Build history of the part. All positions in model axes, mm. A direction names the side the tool comes from. Round coordinates to 2 decimals unless told otherwise and drop trailing zeros. Write each loop counter-clockwise with the first axis right and the second up, starting at its lowest first coordinate (ties: lowest second). Pieces come first, ordered by that corner, then holes. Notation, with made-up numbers: (25.25, -0.75) -> (36.25, -0.75) arc R11 ccw to (36.25, 15.25) -> close; hole circle Ø8 at (83, 35). An arc over 180 degrees is marked (long way). Return JSON: item names as keys, results as strings.
from build123d import *

# Parameters (mm, degrees)
BASE_SKETCH_W                   = 20.493901532
BASE_SKETCH_H                   = 8
BASE_EXTRUDE_DEPTH              = 1.5
PROTRUSION_START                = 1.5
PROTRUSION_SKETCH_R             = 3
PROTRUSION_EXTRUDE_DEPTH        = 5
F_2_8_2_8_DIAMETER_HOLE1_D      = 2.8
PROTRUSION_CHAMFER_SIZE         = 0.25
F_2_5MM_DOWEL_HOLE3_D           = 2.5
F_2_5MM_DOWEL_HOLE3_DEPTH       = 6.5
F_2_5MM_DOWEL_HOLE3_CSINK_D     = 4
F_2_5MM_DOWEL_HOLE3_CSINK_ANGLE = 60
F_5MM_CIRCLE_SKETCH_R           = 2.5
F_5MM_DIAMETER_CUT_DEPTH        = 0.7


with BuildPart() as part:
    # Base Sketch → Base Extrude (new body)
    with BuildSketch(Plane(origin=(0, 0, 0), x_dir=(1, 0, 0), z_dir=(0, 1, 0))):
        with BuildLine():
            Line((-10.246950766, -4), (-10.246950766, 4))
            ThreePointArc((-10.246950766, 4), (-11, 0), (-10.246950766, -4))
        make_face()
        Rectangle(BASE_SKETCH_W, BASE_SKETCH_H)
        with BuildLine():
            Line((10.246950766, -4), (10.246950766, 4))
            ThreePointArc((10.246950766, 4), (11, 0), (10.246950766, -4))
        make_face()
    extrude(amount=BASE_EXTRUDE_DEPTH)

    # Protrusion Sketch → Protrusion Extrude (add)
    with BuildSketch(Plane(origin=(0, 0, 0), x_dir=(1, 0, 0), z_dir=(0, 1, 0)).offset(PROTRUSION_START)):
        Circle(PROTRUSION_SKETCH_R)
    extrude(amount=PROTRUSION_EXTRUDE_DEPTH)

    # Ø2.8 (2.8) Diameter Hole1 (through all)
    with Locations(Plane(origin=(0, 1.5, 0), x_dir=(1, 0, 0), z_dir=(0, 1, 0))):
        with Locations((-6.5, 0), (6.5, 0)):
            Hole(F_2_8_2_8_DIAMETER_HOLE1_D / 2)

    # Protrusion Chamfer
    protrusion_chamfer_edges = [part.edges().sort_by_distance(p)[0] for p in [
        (-3, 6.5, 0),
    ]]
    chamfer(protrusion_chamfer_edges, length=PROTRUSION_CHAMFER_SIZE)

    # Ø2.5mm Dowel Hole3
    with Locations(Plane(origin=(0, 6.5, 0), x_dir=(1, 0, 0), z_dir=(0, 1, 0))):
        with Locations((0, 0)):
            CounterSinkHole(F_2_5MM_DOWEL_HOLE3_D / 2, F_2_5MM_DOWEL_HOLE3_CSINK_D / 2, depth=F_2_5MM_DOWEL_HOLE3_DEPTH, counter_sink_angle=F_2_5MM_DOWEL_HOLE3_CSINK_ANGLE)

    # 5mm Circle Sketch → 5mm Diameter Cut (cut)
    with BuildSketch(Plane(origin=(0, 0, 0), x_dir=(1, 0, 0), z_dir=(0, 1, 0))):
        Circle(F_5MM_CIRCLE_SKETCH_R)
    extrude(amount=F_5MM_DIAMETER_CUT_DEPTH, mode=Mode.SUBTRACT)


solid = part.part
Q1. Saw through at A-A on x = -6.5. List the corners of the cut face in (y, z).
Verdict:
{"outline": "(0, -4) -> (1.5, -4) -> (1.5, -1.4) -> (0, -1.4) -> close; (0, 1.4) -> (1.5, 1.4) -> (1.5, 4) -> (0, 4) -> close"}
Q2. 3-axis set-ups, long thin cutter, end or side, ignore diameter. For faces 1 (the flat face through (-1, 0.7, 1)), 2 (the flat face through (-3, 0, 0)): which of +Z, -Z, +X, -X, +Y, -Y reach the whole face in a straight line?
Verdict:
{"face 1": "-Y", "face 2": "+Z, -Z, +X, -X, -Y"}
Q3. Pin check, flat tips, straight feed: pin 1 Ø1 at (y, z) = (3, -2.5) entering from +X; pin 2 Ø1.5 at (y, z) = (3, 2) entering from +X; pin 3 Ø3 at (y, z) = (1.5, -2) entering from -X. Stop position of each tip, or through.
Verdict:
{"pin 1": "stops at x = 2.24", "pin 2": "stops at x = 2.73", "pin 3": "stops at x = -10.99"}
Q4. Saw through at D-D on x = 0. List the corners of the cut face in (y, z), then the cut area to 3 significant figures.
Verdict:
{"outline": "(0, -4) -> (1.5, -4) -> (1.5, -3) -> (6.25, -3) -> (6.5, -2.75) -> (6.5, -2) -> (5.2, -1.25) -> (0.7, -1.25) -> (0.7, -2.5) -> (0, -2.5) -> close; (0, 2.5) -> (0.7, 2.5) -> (0.7, 1.25) -> (5.2, 1.25) -> (6.5, 2) -> (6.5, 2.75) -> (6.25, 3) -> (1.5, 3) -> (1.5, 4) -> (0, 4) -> close", "area": "23.0 mm²"}
Q5. Saw through at B-B on z = 0. List the corners of the cut face in (x, y), then the cut area to 3 significant figures.
Verdict:
{"outline": "(-11, 0) -> (-7.9, 0) -> (-7.9, 1.5) -> (-11, 1.5) -> close; (-5.1, 0) -> (-2.5, 0) -> (-2.5, 0.7) -> (-1.25, 0.7) -> (-1.25, 5.2) -> (-2, 6.5) -> (-2.75, 6.5) -> (-3, 6.25) -> (-3, 1.5) -> (-5.1, 1.5) -> close; (1.25, 0.7) -> (2.5, 0.7) -> (2.5, 0) -> (5.1, 0) -> (5.1, 1.5) -> (3, 1.5) -> (3, 6.25) -> (2.75, 6.5) -> (2, 6.5) -> (1.25, 5.2) -> close; (7.9, 0) -> (11, 0) -> (11, 1.5) -> (7.9, 1.5) -> close", "area": "35.6 mm²"}
Q6. Saw through at C-C on y = 1.75. List the corners of the cut face in (x, z), then the cut area to 3 significant figures.
Verdict:
{"outline": "circle Ø6 at (0, 0); hole circle Ø2.5 at (0, 0)", "area": "23.4 mm²"}
Q7. Wall check: L1, parallel to Z at x = 0, y = 0.2; L2, parallel to X at y = 1, z = -0.5; L3, parallel to Z at x = 0, y = 3.4. Give the ranges that are in metal, low to high.
Verdict:
{"L1": "z = -4 to -2.5, 2.5 to 4", "L2": "x = -10.99 to -7.81, -5.19 to -1.15, 1.15 to 5.19, 7.81 to 10.99", "L3": "z = -3 to -1.25, 1.25 to 3"}
Q8. Two-plate mould, pull along X, no slides. Class faces 3 (the flat face through (0, 1, 4)), 4 (the cylindrical face through (-3, 4, 0)), 5 (the cylindrical face through (-0.54, 0.35, 2.44)): +X half, -X half, draft (parallel to the pull), parting line (faces both ways), or undercut.
Verdict:
{"face 3": "draft", "face 4": "parting line", "face 5": "undercut"}
